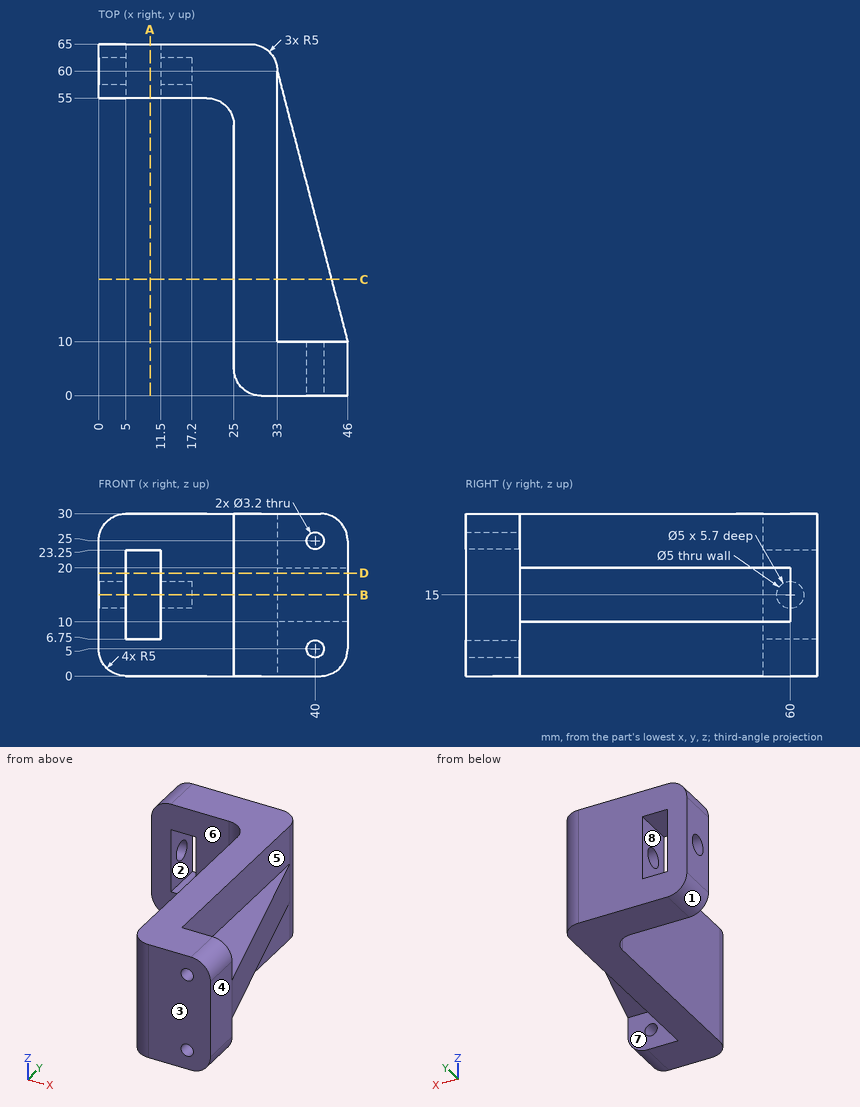
The figure shows three views and two pictorial views of one solid part (mm, origin at its lowest corner). Answer the questions. A direction names the side the tool comes from. Round coordinates to 2 decimals unless told otherwise and drop trailing zeros. Write each loop counter-clockwise with the first axis right and the second up, starting at its lowest first coordinate (ties: lowest second). Pieces come first, ordered by that corner, then holes. Notation, with made-up numbers: (-6, 9) - (35, 9) arc R33 ccw to (35, 47) - close; hole circle Ø5 at (35.25, 20). An arc over 180 degrees is marked (long way). Use one line per item in the form item = value. Start each with the question number.
Item 1: Determine the mould class of the marked faces 1, 2, 3 and 4 for opening direction X: +X half, -X half, draft (parallel to the pull), parting line (faces both ways), or undercut.
Item 2: A cutting plane is placed at B-B (z = 15). Write down the section's boundary in (x, y).
Item 3: A cutting plane is placed at A-A (x = 9.5). Write down the section's boundary in (y, z).
Item 4: Flat-ended cylindrical pins translate along their axes: pin 1 Ø1 at (x, z) = (31, 22.5) entering from +Y; pin 2 Ø3 at (y, z) = (60.5, 17.5) entering from +X; pin 3 Ø10 at (y, z) = (43, 10.5) entering from +X. Find the tip coordinate at first contact, or state that the pin passes through.
Item 5: A cutting plane is placed at D-D (z = 19). Write down the section's boundary in (x, y), plus the area to 3 significant figures.
Item 6: A cutting plane is placed at C-C (y = 21.5). Write down the section's boundary in (x, z), plus the area to 3 significant figures.
Item 7: Find the intervals of material crossed by line 1 (X direction, y = 8, z = 25); line 2 (Y direction, x = 13.8, z = 15); line 3 (X direction, y = 55.5, z = 20.5), in increasing order. Write a range as [from, to].
Item 8: A tool of negligible diameter and unlimited length cuts with its end or side. For the marked faces 5, 6, 7 and 8, from which of +Z, -Z, +X, -X, +Y, -Y can it reach the whole face along a straight path? Write none if from no direction.
The answers:
q1.face_1 = -X half
q1.face_2 = undercut
q1.face_3 = draft
q1.face_4 = +X half
q2.outline = (0, 55) - (5, 55) - (5, 57.5) - (0, 57.5) - close; (0, 62.5) - (5, 62.5) - (5, 65) - (0, 65) - close; (11.5, 55) - (20, 55) arc R5 cw to (25, 50) - (25, 5) arc R5 ccw to (30, 0) - (46, 0) - (46, 10) - (33, 60) arc R5 ccw to (28, 65) - (11.5, 65) - (11.5, 62.5) - (17.2, 62.5) - (17.2, 57.5) - (11.5, 57.5) - close
q3.outline = (55, 0) - (65, 0) - (65, 6.75) - (55, 6.75) - close; (55, 23.25) - (65, 23.25) - (65, 30) - (55, 30) - close
q4.pin_1 = 64.33
q4.pin_2 = 33.26
q4.pin_3 = 38.72
q5.outline = (0, 55) - (5, 55) - (5, 65) - (0, 65) - close; (11.5, 55) - (20, 55) arc R5 cw to (25, 50) - (25, 5) arc R5 ccw to (30, 0) - (46, 0) - (46, 10) - (33, 60) arc R5 ccw to (28, 65) - (11.5, 65) - close
q5.area = 1,150 mm^2
q6.outline = (25, 0) - (33, 0) - (33, 10) - (43.01, 10) - (43.01, 20) - (33, 20) - (33, 30) - (25, 30) - close
q6.area = 340 mm^2
q7.line_1 = [25, 38.4], [41.6, 46]
q7.line_2 = [55, 57.5], [62.5, 65]
q7.line_3 = [0, 5], [11.5, 33]
q8.face_5 = +Z, +X, +Y
q8.face_6 = +Z, -Z, -X, -Y
q8.face_7 = -Z, +X, +Y
q8.face_8 = +Y, -Y
